Read the model definition and answer for the solid it produces. Units are mm, in the model's axes. Coordinates: 2 decimals unless noted, no trailing zeros. Loops run counter-clockwise (first coordinate to the right, second up) from the corner with the lowest first, then second, coordinate; pieces in that order, holes last.
from build123d import *

# Parameters (mm, degrees)
SKETCH_1_R                  = 50
EXTRUDE_1_DEPTH             = 4
CUT_EXTRUDE_2_DEPTH         = 71.823724839
HOLE_WIZARD_M41_D           = 4.5
HOLE_WIZARD_M41_CSINK_D     = 5
HOLE_WIZARD_M41_CSINK_ANGLE = 90
HOLE_WIZARD_M42_D           = 4.5
HOLE_WIZARD_M42_CSINK_D     = 5
HOLE_WIZARD_M42_CSINK_ANGLE = 90


with BuildPart() as part:
    # Эскиз1 → Бобышка-Вытянуть1 (new body)
    with BuildSketch(Plane(origin=(0, 0, 0), x_dir=(1, 0, 0), z_dir=(0, 1, 0))):
        with Locations(Location((0, 0, 0), (0, 0, 270))):
            Circle(SKETCH_1_R)
    extrude(amount=EXTRUDE_1_DEPTH)

    # Эскиз2 → Вырез-Вытянуть2 (cut, through all)
    with BuildSketch(Plane(origin=(0, 0, 0), x_dir=(1, 0, 0), z_dir=(0, 1, 0))):
        with BuildLine():
            Line((8.550503583, -23.49231552), (11.970705016, -32.889241728))
            ThreePointArc((11.970705016, -32.889241728), (17.5, -30.310889132), (22.497566339, -26.811555509))
            Line((22.497566339, -26.811555509), (16.069690242, -19.151111078))
            ThreePointArc((16.069690242, -19.151111078), (12.5, -21.650635095), (8.550503583, -23.49231552))
        make_face()
        with BuildLine():
            Line((-4.341204442, -24.620193825), (-6.077686218, -34.468271355))
            ThreePointArc((-6.077686218, -34.468271355), (0, -35), (6.077686218, -34.468271355))
            Line((6.077686218, -34.468271355), (4.341204442, -24.620193825))
            ThreePointArc((4.341204442, -24.620193825), (0, -25), (-4.341204442, -24.620193825))
        make_face()
        with BuildLine():
            Line((23.49231552, 8.550503583), (32.889241728, 11.970705016))
            ThreePointArc((32.889241728, 11.970705016), (30.310889132, 17.5), (26.811555509, 22.497566339))
            Line((26.811555509, 22.497566339), (19.151111078, 16.069690242))
            ThreePointArc((19.151111078, 16.069690242), (21.650635095, 12.5), (23.49231552, 8.550503583))
        make_face()
        with BuildLine():
            Line((24.620193825, -4.341204442), (34.468271355, -6.077686218))
            ThreePointArc((34.468271355, -6.077686218), (35, 0), (34.468271355, 6.077686218))
            Line((34.468271355, 6.077686218), (24.620193825, 4.341204442))
            ThreePointArc((24.620193825, 4.341204442), (25, 0), (24.620193825, -4.341204442))
        make_face()
        with BuildLine():
            Line((19.151111078, -16.069690242), (26.811555509, -22.497566339))
            ThreePointArc((26.811555509, -22.497566339), (30.310889132, -17.5), (32.889241728, -11.970705016))
            Line((32.889241728, -11.970705016), (23.49231552, -8.550503583))
            ThreePointArc((23.49231552, -8.550503583), (21.650635095, -12.5), (19.151111078, -16.069690242))
        make_face()
        with BuildLine():
            Line((-8.550503583, 23.49231552), (-11.970705016, 32.889241728))
            ThreePointArc((-11.970705016, 32.889241728), (-17.5, 30.310889132), (-22.497566339, 26.811555509))
            Line((-22.497566339, 26.811555509), (-16.069690242, 19.151111078))
            ThreePointArc((-16.069690242, 19.151111078), (-12.5, 21.650635095), (-8.550503583, 23.49231552))
        make_face()
        with BuildLine():
            Line((4.341204442, 24.620193825), (6.077686218, 34.468271355))
            ThreePointArc((6.077686218, 34.468271355), (0, 35), (-6.077686218, 34.468271355))
            Line((-6.077686218, 34.468271355), (-4.341204442, 24.620193825))
            ThreePointArc((-4.341204442, 24.620193825), (0, 25), (4.341204442, 24.620193825))
        make_face()
        with BuildLine():
            Line((16.069690242, 19.151111078), (22.497566339, 26.811555509))
            ThreePointArc((22.497566339, 26.811555509), (17.5, 30.310889132), (11.970705016, 32.889241728))
            Line((11.970705016, 32.889241728), (8.550503583, 23.49231552))
            ThreePointArc((8.550503583, 23.49231552), (12.5, 21.650635095), (16.069690242, 19.151111078))
        make_face()
        with BuildLine():
            Line((-16.069690242, -19.151111078), (-22.497566339, -26.811555509))
            ThreePointArc((-22.497566339, -26.811555509), (-17.5, -30.310889132), (-11.970705016, -32.889241728))
            Line((-11.970705016, -32.889241728), (-8.550503583, -23.49231552))
            ThreePointArc((-8.550503583, -23.49231552), (-12.5, -21.650635095), (-16.069690242, -19.151111078))
        make_face()
        with BuildLine():
            Line((-23.49231552, -8.550503583), (-32.889241728, -11.970705016))
            ThreePointArc((-32.889241728, -11.970705016), (-30.310889132, -17.5), (-26.811555509, -22.497566339))
            Line((-26.811555509, -22.497566339), (-19.151111078, -16.069690242))
            ThreePointArc((-19.151111078, -16.069690242), (-21.650635095, -12.5), (-23.49231552, -8.550503583))
        make_face()
        with BuildLine():
            Line((-24.620193825, 4.341204442), (-34.468271355, 6.077686218))
            ThreePointArc((-34.468271355, 6.077686218), (-35, 0), (-34.468271355, -6.077686218))
            Line((-34.468271355, -6.077686218), (-24.620193825, -4.341204442))
            ThreePointArc((-24.620193825, -4.341204442), (-25, 0), (-24.620193825, 4.341204442))
        make_face()
        with BuildLine():
            Line((-19.151111078, 16.069690242), (-26.811555509, 22.497566339))
            ThreePointArc((-26.811555509, 22.497566339), (-30.310889132, 17.5), (-32.889241728, 11.970705016))
            Line((-32.889241728, 11.970705016), (-23.49231552, 8.550503583))
            ThreePointArc((-23.49231552, 8.550503583), (-21.650635095, 12.5), (-19.151111078, 16.069690242))
        make_face()
    extrude(amount=CUT_EXTRUDE_2_DEPTH, mode=Mode.SUBTRACT)

    # Отверстие с зазором M41 (through all)
    with Locations(Plane(origin=(0, 0, 0), x_dir=(-1, 0, 0), z_dir=(0, -1, 0))):
        with Locations((0, 42.5), (21.25, 36.806079661), (36.806079661, 21.25), (42.5, 0), (36.806079661, -21.25), (21.25, -36.806079661), (0, -42.5), (-21.25, -36.806079661), (-36.806079661, -21.25), (-42.5, 0), (-36.806079661, 21.25), (-21.25, 36.806079661)):
            CounterSinkHole(HOLE_WIZARD_M41_D / 2, HOLE_WIZARD_M41_CSINK_D / 2, counter_sink_angle=HOLE_WIZARD_M41_CSINK_ANGLE)

    # Отверстие с зазором M42 (through all)
    with Locations(Plane(origin=(0, 4, 0), x_dir=(1, 0, 0), z_dir=(0, 1, 0))):
        with Locations((-17.320508076, 10), (0, 20), (17.320508076, 10), (17.320508076, -10), (0, -20), (-17.320508076, -10)):
            CounterSinkHole(HOLE_WIZARD_M42_D / 2, HOLE_WIZARD_M42_CSINK_D / 2, counter_sink_angle=HOLE_WIZARD_M42_CSINK_ANGLE)


solid = part.part
Item 1: A cutting plane is placed at B-B on x = 21.25. Give the number of separate pieces and of enclosed holes in the cut face, then the cut area to 3 significant figures.
Numbers:
separate pieces: 7
enclosed holes: 0
area: 269 mm2
Item 2: A cutting plane is placed at C-C on z = -10. Determine the outline of the cut face in (x, y), then the cut area to 3 significant figures.
Numbers:
outline: (-48.99, 0) - (-27.47, 0) - (-27.47, 4) - (-48.99, 4) - close; (-22.91, 0) - (-19.57, 0) - (-19.57, 3.75) - (-19.82, 4) - (-22.91, 4) - close; (-15.07, 0) - (15.07, 0) - (15.07, 3.75) - (14.82, 4) - (-14.82, 4) - (-15.07, 3.75) - close; (19.57, 0) - (22.91, 0) - (22.91, 4) - (19.82, 4) - (19.57, 3.75) - close; (27.47, 0) - (48.99, 0) - (48.99, 4) - (27.47, 4) - close
area: 319 mm2
Item 3: A cutting plane is placed at A-A on z = 42.5. Determine the outline of the cut face in (x, y), then the cut area to 3 significant figures.
Numbers:
outline: (-26.34, 0) - (-2.5, 0) - (-2.25, 0.25) - (-2.25, 4) - (-26.34, 4) - close; (2.25, 0.25) - (2.5, 0) - (26.34, 0) - (26.34, 4) - (2.25, 4) - close
area: 193 mm2
Item 4: A cutting plane is placed at D-D on x = 42.5. Determine the outline of the cut face in (y, z), then the cut area to 3 significant figures.
Numbers:
outline: (0, -26.34) - (4, -26.34) - (4, -2.25) - (0.25, -2.25) - (0, -2.5) - close; (0, 2.5) - (0.25, 2.25) - (4, 2.25) - (4, 26.34) - (0, 26.34) - close
area: 193 mm2
Item 5: Determine the mould class of faces 1 (the face through (-20.21, 2.15, -34.81)), 2 (the face through (0.488, 1.849, 22.196)) for opening direction X: released by +X, released by -X, zero draft, split by the parting line, or undercut.
Numbers:
face 1: undercut
face 2: undercut
Item 6: Given pin 1 (5 mm diameter, centred on x = 0, z = -20, fed in from -Y); pin 2 (1 mm diameter, centred on y = 1, z = -9, fed in from -X); pin 3 (1.5 mm diameter, centred on y = 2, z = 38.5, fed in from -X), each flat-ended and moving along its own axis, determine where each tip first touches the part or whether it passes through.
Numbers:
pin 1: stops at y = 0
pin 2: stops at x = -49.27
pin 3: stops at x = -32.79
Item 7: Find the intervals of material crossed by line 1 along Z through (x, y) = (-15.5, 2.85); line 2 along X through (y, z) = (0.2, -4); line 3 along Z through (x, y) = (-32, 1.45), in increasing order.
Numbers:
line 1: z = -47.54 to -31.38, -19.62 to -11.32, -8.68 to 8.68, 11.32 to 19.62, 31.38 to 47.54
line 2: x = -49.84 to -34.77, -24.68 to 24.68, 34.77 to 49.84
line 3: z = -38.42 to -14.18, -11.65 to -5.64, 5.64 to 11.65, 14.18 to 38.42
